For this review, take the finished solid that the model builds, in its own axes (mm). A direction names the side the tool comes from. Round coordinates to 2 decimals unless told otherwise and drop trailing zeros. Order: outer loops, then holes, each group sorted by start corner. A loop starts at its lowest first (then second) coordinate and runs counter-clockwise, first axis right, second up. Notation, with made-up numbers: M 26,46 L 85,46 A14 ccw 85,58 Z; hole C 56,-10.5 d10. An arc over 180 degrees is marked long. Put each result on its own line as item: value.
from build123d import *

# Parameters (mm, degrees)
CYLINDER008_R     = 8.25
CYLINDER008_DEPTH = 30
BOX008_W          = 3.2
BOX008_H          = 90
BOX008_DEPTH      = 4
BOX006_W          = 3.2
BOX006_H          = 90
BOX006_DEPTH      = 4
BOX004_W          = 3.2
BOX004_H          = 90
BOX004_DEPTH      = 4
CYLINDER007_R     = 4
CYLINDER007_DEPTH = 25
CYLINDER006_R     = 4
CYLINDER006_DEPTH = 25
CYLINDER005_R     = 4
CYLINDER005_DEPTH = 25
CYLINDER004_R     = 4
CYLINDER004_DEPTH = 25
CYLINDER003_R     = 6.05
CYLINDER003_DEPTH = 25
CYLINDER002_R     = 6.05
CYLINDER002_DEPTH = 25
CYLINDER001_R     = 6.05
CYLINDER001_DEPTH = 25
CYLINDER_R        = 6.05
CYLINDER_DEPTH    = 25
BOX001_W          = 40
BOX001_H          = 55
BOX001_DEPTH      = 7
BOX_W             = 36.8
BOX_H             = 85
BOX_DEPTH         = 30


with BuildPart() as cylinder008:
    # Cylinder008 → Cylinder008 (new body)
    with BuildSketch(Plane(origin=(17, 45, 5), x_dir=(1, 0, 0), z_dir=(0, 0, 1))):
        Circle(CYLINDER008_R)
    extrude(amount=CYLINDER008_DEPTH)


with BuildPart() as cube008:
    # Box008 → Box008 (new body)
    with BuildSketch(Plane(origin=(28.4, -3, 0), x_dir=(1, 0, 0), z_dir=(0, 0, 1))):
        with Locations((1.6, 45)):
            Rectangle(BOX008_W, BOX008_H)
    extrude(amount=BOX008_DEPTH)


with BuildPart() as cube006:
    # Box006 → Box006 (new body)
    with BuildSketch(Plane(origin=(17.2, -3, 0), x_dir=(1, 0, 0), z_dir=(0, 0, 1))):
        with Locations((1.6, 45)):
            Rectangle(BOX006_W, BOX006_H)
    extrude(amount=BOX006_DEPTH)


with BuildPart() as cube004:
    # Box004 → Box004 (new body)
    with BuildSketch(Plane(origin=(6, -3, 0), x_dir=(1, 0, 0), z_dir=(0, 0, 1))):
        with Locations((1.6, 45)):
            Rectangle(BOX004_W, BOX004_H)
    extrude(amount=BOX004_DEPTH)


with BuildPart() as cylinder007:
    # Cylinder007 → Cylinder007 (new body)
    with BuildSketch(Plane(origin=(6.5, 61.5, 5), x_dir=(1, 0, 0), z_dir=(0, 0, 1))):
        Circle(CYLINDER007_R)
    extrude(amount=CYLINDER007_DEPTH)


with BuildPart() as cylinder006:
    # Cylinder006 → Cylinder006 (new body)
    with BuildSketch(Plane(origin=(30.5, 75, 5), x_dir=(1, 0, 0), z_dir=(0, 0, 1))):
        Circle(CYLINDER006_R)
    extrude(amount=CYLINDER006_DEPTH)


with BuildPart() as cylinder005:
    # Cylinder005 → Cylinder005 (new body)
    with BuildSketch(Plane(origin=(27.5, 61.5, 5), x_dir=(1, 0, 0), z_dir=(0, 0, 1))):
        Circle(CYLINDER005_R)
    extrude(amount=CYLINDER005_DEPTH)


with BuildPart() as cylinder004:
    # Cylinder004 → Cylinder004 (new body)
    with BuildSketch(Plane(origin=(12.5, 75, 5), x_dir=(1, 0, 0), z_dir=(0, 0, 1))):
        Circle(CYLINDER004_R)
    extrude(amount=CYLINDER004_DEPTH)


with BuildPart() as cylinder003:
    # Cylinder003 → Cylinder003 (new body)
    with BuildSketch(Plane(origin=(27.5, 23.5, 5), x_dir=(1, 0, 0), z_dir=(0, 0, 1))):
        Circle(CYLINDER003_R)
    extrude(amount=CYLINDER003_DEPTH)


with BuildPart() as cylinder002:
    # Cylinder002 → Cylinder002 (new body)
    with BuildSketch(Plane(origin=(9.5, 23.5, 5), x_dir=(1, 0, 0), z_dir=(0, 0, 1))):
        Circle(CYLINDER002_R)
    extrude(amount=CYLINDER002_DEPTH)


with BuildPart() as cylinder001:
    # Cylinder001 → Cylinder001 (new body)
    with BuildSketch(Plane(origin=(27.5, 6, 5), x_dir=(1, 0, 0), z_dir=(0, 0, 1))):
        Circle(CYLINDER001_R)
    extrude(amount=CYLINDER001_DEPTH)


with BuildPart() as cylinder:
    # Cylinder → Cylinder (new body)
    with BuildSketch(Plane(origin=(9.5, 6, 5), x_dir=(1, 0, 0), z_dir=(0, 0, 1))):
        Circle(CYLINDER_R)
    extrude(amount=CYLINDER_DEPTH)


with BuildPart() as cube001:
    # Box001 → Box001 (new body)
    with BuildSketch(Plane(origin=(0, 33, 23), x_dir=(1, 0, 0), z_dir=(0, 0, 1))):
        with Locations((20, 27.5)):
            Rectangle(BOX001_W, BOX001_H)
    extrude(amount=BOX001_DEPTH)


with BuildPart() as cut012:
    # Box → Box (new body)
    with BuildSketch(Plane(origin=(0, -3, 0), x_dir=(1, 0, 0), z_dir=(0, 0, 1))):
        with Locations((18.4, 42.5)):
            Rectangle(BOX_W, BOX_H)
    extrude(amount=BOX_DEPTH)

    # Cut: cut Cube001
    add(cube001.part, mode=Mode.SUBTRACT)

    # Cut001: cut Cylinder
    add(cylinder.part, mode=Mode.SUBTRACT)

    # Cut002: cut Cylinder001
    add(cylinder001.part, mode=Mode.SUBTRACT)

    # Cut003: cut Cylinder002
    add(cylinder002.part, mode=Mode.SUBTRACT)

    # Cut004: cut Cylinder003
    add(cylinder003.part, mode=Mode.SUBTRACT)

    # Cut005: cut Cylinder004
    add(cylinder004.part, mode=Mode.SUBTRACT)

    # Cut006: cut Cylinder005
    add(cylinder005.part, mode=Mode.SUBTRACT)

    # Cut007: cut Cylinder006
    add(cylinder006.part, mode=Mode.SUBTRACT)

    # Cut008: cut Cylinder007
    add(cylinder007.part, mode=Mode.SUBTRACT)

    # Cut009: cut Cube004
    add(cube004.part, mode=Mode.SUBTRACT)

    # Cut010: cut Cube006
    add(cube006.part, mode=Mode.SUBTRACT)

    # Cut011: cut Cube008
    add(cube008.part, mode=Mode.SUBTRACT)

    # Cut012: cut Cylinder008
    add(cylinder008.part, mode=Mode.SUBTRACT)


solid = cut012.part
(1) Add section A-A on y = 45. Give the boundary of the cut face in (x, z).
A:
outline: M 0,0 L 6,0 L 6,4 L 9.2,4 L 9.2,0 L 17.2,0 L 17.2,4 L 20.4,4 L 20.4,0 L 28.4,0 L 28.4,4 L 31.6,4 L 31.6,0 L 36.8,0 L 36.8,23 L 25.25,23 L 25.25,5 L 8.75,5 L 8.75,23 L 0,23 Z
(2) Add section C-C on y = 55. Give the boundary of the cut face in (x, z).
A:
outline: M 0,0 L 6,0 L 6,4 L 9.2,4 L 9.2,0 L 17.2,0 L 17.2,4 L 20.4,4 L 20.4,0 L 28.4,0 L 28.4,4 L 31.6,4 L 31.6,0 L 36.8,0 L 36.8,23 L 0,23 Z
(3) Draft analysis for pull direction Y (two halves, no side actions). For faces 4 (the face through (3, 40, 0)), 5 (the face through (3.456, 6.266, 17.325)), 6 (the face through (18, -3, 15)), state which applies: released by +Y, released by -Y, zero draft, split by the parting line, or undercut.
A:
face 4: zero draft
face 5: undercut
face 6: released by -Y
(4) Add section B-B on x = 13.5. Give the boundary of the cut face in (y, z), then the cut area to 3 significant figures.
A:
outline: M -3,0 L 82,0 L 82,23 L 78.87,23 L 78.87,5 L 71.13,5 L 71.13,23 L 52.47,23 L 52.47,5 L 37.53,5 L 37.53,23 L 33,23 L 33,30 L 28.04,30 L 28.04,5 L 18.96,5 L 18.96,30 L 10.54,30 L 10.54,5 L 1.46,5 L 1.46,30 L -3,30 Z
area: 1,340 mm2
(5) Add section D-D on x = 5. Give the boundary of the cut face in (y, z).
A:
outline: M -3,0 L 82,0 L 82,23 L 65.21,23 L 65.21,5 L 57.79,5 L 57.79,23 L 33,23 L 33,30 L 27.54,30 L 27.54,5 L 19.46,5 L 19.46,30 L 10.04,30 L 10.04,5 L 1.96,5 L 1.96,30 L -3,30 Z
(6) Insertion check: pin 1 Ø13 at (x, y) = (6.5, 61.5) entering from +Z; pin 2 Ø6 at (x, y) = (26.5, 25.5) entering from +Z; pin 3 Ø1 at (x, y) = (19, 37.5) entering from -Z. Each pin has a flat end and moves straight along its axis. Give the tip position at first contact, or say it passes through.
A:
pin 1: stops at z = 23
pin 2: stops at z = 5
pin 3: stops at z = 4
(7) To check wall thickness, follow L1, parallel to X at y = 15.5, z = 2.5; L2, parallel to X at y = 75, z = 10; L3, parallel to Y at x = 12.5, z = 17.5. State the ranges of each line that lie inside material, in increasing order.
A:
L1: x = 0 to 6, 9.2 to 17.2, 20.4 to 28.4, 31.6 to 36.8
L2: x = 0 to 8.5, 16.5 to 26.5, 34.5 to 36.8
L3: y = -3 to 0.75, 11.25 to 18.25, 28.75 to 38.09, 51.91 to 71, 79 to 82
(8) For faces 1 (the face through (20.4, 39, 2)), 2 (the face through (29.633, 71.095, 13.874)), 3 (the face through (24, 40, 0)), list the 3-axis set-ups (+Z, -Z, +X, -X, +Y, -Y) from which the entire face can be reached by the end or side of a thin tool; tool diameter is ignored.
A:
face 1: -Z, +Y, -Y
face 2: +Z
face 3: -Z, +X, -X, +Y, -Y
